```python
from build123d import *

# Parameters (mm, degrees)
SALIENTE_EXTRUIR1_DEPTH = 10
CROQUIS4_W              = 2
CROQUIS4_H              = 6
SALIENTE_EXTRUIR2_DEPTH = 10
CROQUIS5_R              = 1.625
CORTAR_EXTRUIR1_DEPTH   = 4


with BuildPart() as part:
    # Croquis2 → Saliente-Extruir1 (new body)
    with BuildSketch(Plane(origin=(0, 0, 0), x_dir=(0, 0, -1), z_dir=(1, 0, 0))):
        Polygon((0, 0), (13, 0), (13, 9.8), (25.65, 9.8), (25.65, 12.8), (10, 12.8), (10, 3), (0, 3), align=None)
    extrude(amount=SALIENTE_EXTRUIR1_DEPTH)

    # Croquis4 → Saliente-Extruir2 (add, through all)
    with BuildSketch(Plane(origin=(0, 0, 0), x_dir=(0, 0, -1), z_dir=(1, 0, 0))):
        with Locations((26.65, 9.8)):
            Rectangle(CROQUIS4_W, CROQUIS4_H)
    extrude(amount=SALIENTE_EXTRUIR2_DEPTH)

    # Croquis5 → Cortar-Extruir1 (cut, through all)
    with BuildSketch(Plane(origin=(0, 3, 0), x_dir=(1, 0, 0), z_dir=(0, 1, 0))):
        with Locations((5, 5)):
            Circle(CROQUIS5_R)
    extrude(amount=-CORTAR_EXTRUIR1_DEPTH, mode=Mode.SUBTRACT)


solid = part.part
```
Geometry check sheet. Reference: the model listing, model coordinates, mm. A direction names the side the tool comes from. Coordinates: 2 decimals unless noted, no trailing zeros. Write each loop counter-clockwise with the first axis right and the second up, starting at its lowest first coordinate (ties: lowest second). Pieces come first, ordered by that corner, then holes. Notation, with made-up numbers: M 14,48 L 58,48 A11 cw 58,61 Z; hole C 19.25,-35.75 d3. An arc over 180 degrees is marked long. Use one line per item in the form item = value. Start each with the question number.
1) Section check C-C on x = 5. Enter the section's corners in (y, z) (3 decimals).
2) Release check for a two-part mould opening along Z. For faces 4 (the flat face through (5, 8, -10)), 5 (the cylindrical face through (3.377, 1.521, -5.071)), 6 (the flat face through (5, 6.8, -27)) record: pulls with the +Z half, pulls with the -Z half, needs draft (parallel to the pull), parting line crosses it, or undercut.
3) Section check D-D on x = 1.75. Enter the section's corners in (y, z), and give its area (3 significant figures).
4) Set-up check for faces 1 (the flat face through (3, 3, -5)), 2 (the flat face through (5, 9.8, -19)), 3 (the flat face through (10, 6.9, -12.7)): record each of +Z, -Z, +X, -X, +Y, -Y from which the full face is reachable in a straight line by a thin tool's end or side.
5) Thickness scan on probe 1 along X at (y, z) = (1.05, -5) (3 decimals); probe 2 along Z at (x, y) = (5, 2.25) (3 decimals); probe 3 along Z at (x, y) = (9, 9). Record the ranges inside material, lowest first. Write a range as from..to.
6) Go/stop test with flat-tipped pins: pin 1 Ø6 at (x, z) = (7, -4.5) entering from +Y; pin 2 Ø0.6 at (x, z) = (5.5, -27) entering from -Y; pin 3 Ø6 at (x, y) = (7, 1.5) entering from -Z. Record where each tip stops, or that it passes through.
7) Section check A-A on y = 8.75. Enter the section's corners in (x, z).
8) Section check B-B on z = -5. Enter the section's corners in (x, y) (3 decimals).
Responses:
q1.outline = M 0,-13 L 9.8,-13 L 9.8,-25.65 L 6.8,-25.65 L 6.8,-27.65 L 12.8,-27.65 L 12.8,-10 L 3,-10 L 3,-6.625 L 0,-6.625 Z; M 0,-3.375 L 3,-3.375 L 3,0 L 0,0 Z
q2.face_4 = pulls with the +Z half
q2.face_5 = undercut
q2.face_6 = needs draft
q3.outline = M 0,-13 L 9.8,-13 L 9.8,-25.65 L 6.8,-25.65 L 6.8,-27.65 L 12.8,-27.65 L 12.8,-10 L 3,-10 L 3,0 L 0,0 Z
q3.area = 118 mm2
q4.face_1 = +Z, +X, -X, +Y
q4.face_2 = +X, -X, -Y
q4.face_3 = +Z, -Z, +X, +Y, -Y
q5.probe_1 = 0..3.375, 6.625..10
q5.probe_2 = -13..-6.625, -3.375..0
q5.probe_3 = -27.65..-25.65, -13..-10
q6.pin_1 = 3
q6.pin_2 = 6.8
q6.pin_3 = -13
q7.outline = M 0,-27.65 L 10,-27.65 L 10,-25.65 L 0,-25.65 Z; M 0,-13 L 10,-13 L 10,-10 L 0,-10 Z
q8.outline = M 0,0 L 3.375,0 L 3.375,3 L 0,3 Z; M 6.625,0 L 10,0 L 10,3 L 6.625,3 Z
